The listing builds one solid part. Answer for the finished solid, in the listing's coordinates (mm). A direction names the side the tool comes from. Coordinates: 2 decimals unless noted, no trailing zeros. Order: outer loops, then holes, each group sorted by start corner. A loop starts at its lowest first (then second) coordinate and runs counter-clockwise, first axis right, second up.
```python
from build123d import *

# Parameters (mm, degrees)
ESQUISSE1_R                    = 1.25
ESQUISSE1_R_2                  = 5
BOSS_EXTRU_1_DEPTH             = 7.5
BOSS_EXTRU_2_DEPTH             = 40
BOSS_EXTRU_2_DIRECTION_2_REACH = 95.383
ESQUISSE4_W                    = 18
ESQUISSE4_H                    = 12.605144054
ENL_V_MAT_EXTRU_1_DEPTH        = 10
ENL_V_START                    = -7.5
ENL_V_MAT_EXTRU_2_DEPTH        = 7.5
BOSS_EXTRU_3_START             = -4
BOSS_EXTRU_3_DEPTH             = 4
BOSS_EXTRU_4_START             = -2
BOSS_EXTRU_4_DEPTH             = 2
ESQUISSE6_R                    = 1.5
ENL_V_MAT_EXTRU_3_DEPTH        = 10
ESQUISSE7_R                    = 3.1
ENL_V_MAT_EXTRU_4_DEPTH        = 2.5
ESQUISSE8_R                    = 3.6
ENL_V_MAT_EXTRU_5_DEPTH        = 0.7


with BuildPart() as part:
    # Esquisse1 → Boss.-Extru.1 (new body)
    with BuildSketch(Plane.XY):
        with BuildLine():
            ThreePointArc((23.75, 0), (0, 23.75), (-23.75, 0))
            Line((-23.75, 0), (-15, -75))
            ThreePointArc((-15, -75), (0, -90), (15, -75))
            Line((15, -75), (23.75, 0))
        make_face()
        with Locations((-5, 5)):
            Circle(ESQUISSE1_R, mode=Mode.SUBTRACT)
        with Locations((5, 5)):
            Circle(ESQUISSE1_R, mode=Mode.SUBTRACT)
        with Locations((5, -5)):
            Circle(ESQUISSE1_R, mode=Mode.SUBTRACT)
        with Locations((-5, -5)):
            Circle(ESQUISSE1_R, mode=Mode.SUBTRACT)
        with Locations((0, -75)):
            Circle(ESQUISSE1_R_2, mode=Mode.SUBTRACT)
    extrude(amount=BOSS_EXTRU_1_DEPTH)

    # Esquisse2 → Boss.-Extru.2 (add)
    with BuildSketch(Plane.XY.offset(7.5)):
        with BuildLine():
            ThreePointArc((-23.75, 0), (0, 23.75), (23.75, 0))
            Line((23.75, 0), (21.125, -22.5))
            Line((21.125, -22.5), (24.145347662, -22.5))
            Line((24.145347662, -22.5), (26.749397242, -0.17957503))
            ThreePointArc((26.749397242, -0.17957503), (0, 26.75), (-26.749397242, -0.17957503))
            Line((-26.749397242, -0.17957503), (-24.145347662, -22.5))
            Line((-24.145347662, -22.5), (-21.125, -22.5))
            Line((-21.125, -22.5), (-23.75, 0))
        make_face()
    extrude(amount=BOSS_EXTRU_2_DEPTH)

    # Boss.-Extru.2 direction 2: up to this face of the body (flat: up to its plane)
    boss_extru_2_direction_2_end = Plane(part.part.faces().sort_by_distance((0, -28.342449308, 0))[0])
    # Esquisse2 → Boss.-Extru.2 direction 2 (add, up to the picked face)
    with BuildSketch(Plane.XY.offset(7.5), mode=Mode.PRIVATE) as boss_extru_2_direction_2_sk1:
        with BuildLine():
            ThreePointArc((-23.75, 0), (0, 23.75), (23.75, 0))
            Line((23.75, 0), (21.125, -22.5))
            Line((21.125, -22.5), (24.145347662, -22.5))
            Line((24.145347662, -22.5), (26.749397242, -0.17957503))
            ThreePointArc((26.749397242, -0.17957503), (0, 26.75), (-26.749397242, -0.17957503))
            Line((-26.749397242, -0.17957503), (-24.145347662, -22.5))
            Line((-24.145347662, -22.5), (-21.125, -22.5))
            Line((-21.125, -22.5), (-23.75, 0))
        make_face()
    boss_extru_2_direction_2_tool1 = split(extrude(boss_extru_2_direction_2_sk1.sketch, amount=-BOSS_EXTRU_2_DIRECTION_2_REACH, mode=Mode.PRIVATE), bisect_by=boss_extru_2_direction_2_end, keep=Keep.BOTH, mode=Mode.PRIVATE)
    add(boss_extru_2_direction_2_tool1.solids().sort_by(Axis((0, 24.477173, 7.5), (0, 0, -1)))[0])

    # Esquisse4 → Enlèv. mat.-Extru.1 (cut)
    with BuildSketch(Plane.XY.offset(47.5)):
        with Locations((0, 26.75)):
            Rectangle(ESQUISSE4_W, ESQUISSE4_H)
    extrude(amount=-ENL_V_MAT_EXTRU_1_DEPTH, mode=Mode.SUBTRACT)

    # Esquisse5 → Enlèv. mat.-Extru.2 (cut)
    with BuildSketch(Plane.XY.offset(47.5).offset(ENL_V_START)):
        with BuildLine():
            Line((-11.411137634, 20.829028732), (-11.640060124, 21.354079473))
            Line((-11.640060124, 21.354079473), (-14.50858003, 21.678003669))
            Line((-14.50858003, 21.678003669), (-16.223366565, 19.355754657))
            Line((-16.223366565, 19.355754657), (-15.594359578, 17.913080398))
            ThreePointArc((-15.594359578, 17.913080398), (-13.581233692, 19.483649335), (-11.411137634, 20.829028732))
        make_face()
        Polygon((-21.820839715, -16.535659582), (-22.588746921, -16.571688322), (-23.913370218, -19.136587239), (-22.354414246, -21.566194123), (-21.240043834, -21.513909991), align=None)
    enl_v_mat_extru_2 = extrude(amount=ENL_V_MAT_EXTRU_2_DEPTH, mode=Mode.SUBTRACT)

    # Esquisse5<3> → Boss.-Extru.3 (add)
    with BuildSketch(Plane.XY.offset(47.5).offset(BOSS_EXTRU_3_START)):
        with BuildLine():
            ThreePointArc((-10.635661114, 21.235470625), (-11.025272446, 21.035823433), (-11.411137634, 20.829028732))
            Line((-11.411137634, 20.829028732), (-10.486326754, 18.707906265))
            Line((-10.486326754, 18.707906265), (-12.201113289, 16.385657254))
            Line((-12.201113289, 16.385657254), (-15.069633195, 16.70958145))
            Line((-15.069633195, 16.70958145), (-15.594359578, 17.913080398))
            ThreePointArc((-15.594359578, 17.913080398), (-15.976876587, 17.572760584), (-16.351968659, 17.224274178))
            ThreePointArc((-16.351968659, 17.224274178), (-12.416744053, 15.659892813), (-9.854846659, 19.031830461))
            ThreePointArc((-9.854846659, 19.031830461), (-10.055820333, 20.200772417), (-10.635661114, 21.235470625))
        make_face()
        with BuildLine():
            ThreePointArc((-17.529790949, -19.001295206), (-18.895919972, -16.227021489), (-21.927845037, -15.618471111))
            Line((-21.927845037, -15.618471111), (-21.820839715, -16.535659582))
            Line((-21.820839715, -16.535659582), (-19.705167652, -16.436396289))
            Line((-19.705167652, -16.436396289), (-18.14621168, -18.866003173))
            Line((-18.14621168, -18.866003173), (-19.470834977, -21.43090209))
            Line((-19.470834977, -21.43090209), (-21.240043834, -21.513909991))
            Line((-21.240043834, -21.513909991), (-21.125, -22.5))
            ThreePointArc((-21.125, -22.5), (-18.588810785, -21.509604565), (-17.529790949, -19.001295206))
        make_face()
    boss_extru_3 = extrude(amount=BOSS_EXTRU_3_DEPTH)

    # Esquisse5<4> → Boss.-Extru.4 (add)
    with BuildSketch(Plane.XY.offset(47.5).offset(BOSS_EXTRU_4_START)):
        with BuildLine():
            Line((-11.411137634, 20.829028732), (-11.640060124, 21.354079473))
            Line((-11.640060124, 21.354079473), (-14.50858003, 21.678003669))
            Line((-14.50858003, 21.678003669), (-16.223366565, 19.355754657))
            Line((-16.223366565, 19.355754657), (-15.594359578, 17.913080398))
            ThreePointArc((-15.594359578, 17.913080398), (-15.089714795, 18.340201945), (-14.573376801, 18.753111438))
            ThreePointArc((-14.573376801, 18.753111438), (-14.072849168, 20.055047153), (-12.678292605, 20.082913051))
            ThreePointArc((-12.678292605, 20.082913051), (-12.050491046, 20.465780355), (-11.411137634, 20.829028732))
        make_face()
        with BuildLine():
            Line((-10.486326754, 18.707906265), (-11.411137634, 20.829028732))
            ThreePointArc((-11.411137634, 20.829028732), (-12.050491046, 20.465780355), (-12.678292605, 20.082913051))
            ThreePointArc((-12.678292605, 20.082913051), (-12.257533448, 19.630498747), (-12.104846659, 19.031830461))
            ThreePointArc((-12.104846659, 19.031830461), (-13.214601654, 17.789722842), (-14.573376801, 18.753111438))
            ThreePointArc((-14.573376801, 18.753111438), (-15.089714795, 18.340201945), (-15.594359578, 17.913080398))
            Line((-15.594359578, 17.913080398), (-15.069633195, 16.70958145))
            Line((-15.069633195, 16.70958145), (-12.201113289, 16.385657254))
            Line((-12.201113289, 16.385657254), (-10.486326754, 18.707906265))
        make_face()
        with BuildLine():
            Line((-19.705167652, -16.436396289), (-21.820839715, -16.535659582))
            Line((-21.820839715, -16.535659582), (-21.659180538, -17.921309676))
            ThreePointArc((-21.659180538, -17.921309676), (-20.406989611, -17.917497027), (-19.779790949, -19.001295206))
            ThreePointArc((-19.779790949, -19.001295206), (-20.285594046, -20.005621333), (-21.393664499, -20.197161436))
            Line((-21.393664499, -20.197161436), (-21.240043834, -21.513909991))
            Line((-21.240043834, -21.513909991), (-19.470834977, -21.43090209))
            Line((-19.470834977, -21.43090209), (-18.14621168, -18.866003173))
            Line((-18.14621168, -18.866003173), (-19.705167652, -16.436396289))
        make_face()
        with BuildLine():
            Line((-21.659180538, -17.921309676), (-21.820839715, -16.535659582))
            Line((-21.820839715, -16.535659582), (-22.588746921, -16.571688322))
            Line((-22.588746921, -16.571688322), (-23.913370218, -19.136587239))
            Line((-23.913370218, -19.136587239), (-22.354414246, -21.566194123))
            Line((-22.354414246, -21.566194123), (-21.240043834, -21.513909991))
            Line((-21.240043834, -21.513909991), (-21.393664499, -20.197161436))
            ThreePointArc((-21.393664499, -20.197161436), (-22.271369873, -19.14614608), (-21.659180538, -17.921309676))
        make_face()
    boss_extru_4 = extrude(amount=BOSS_EXTRU_4_DEPTH)

    # Symétrie1: Enlèv. mat.-Extru.2, Boss.-Extru.3, Boss.-Extru.4 across plane
    add(enl_v_mat_extru_2.mirror(Plane(origin=(0, 0, 0), x_dir=(0, 0, 1), z_dir=(1, 0, 0))), mode=Mode.SUBTRACT)
    add(boss_extru_3.mirror(Plane(origin=(0, 0, 0), x_dir=(0, 0, 1), z_dir=(1, 0, 0))))
    add(boss_extru_4.mirror(Plane(origin=(0, 0, 0), x_dir=(0, 0, 1), z_dir=(1, 0, 0))))

    # Esquisse6 → Enlèv. mat.-Extru.3 (cut)
    with BuildSketch(Plane.XY.offset(7.5)):
        Circle(ESQUISSE6_R)
    extrude(amount=-ENL_V_MAT_EXTRU_3_DEPTH, mode=Mode.SUBTRACT)

    # Esquisse7 → Enlèv. mat.-Extru.4 (cut)
    with BuildSketch(Plane.XY.offset(7.5)):
        Circle(ESQUISSE7_R)
    extrude(amount=-ENL_V_MAT_EXTRU_4_DEPTH, mode=Mode.SUBTRACT)

    # Esquisse8 → Enlèv. mat.-Extru.5 (cut)
    with BuildSketch(Plane.XY.offset(7.5)):
        Circle(ESQUISSE8_R)
    extrude(amount=-ENL_V_MAT_EXTRU_5_DEPTH, mode=Mode.SUBTRACT)


solid = part.part
```
(1) Find section A-A (x = 0). Write down the section's boundary in (y, z), and give its area (3 significant figures).
(2) For faces 1 (the face through (3.434, 1.081, 7.155)), 2 (the face through (-9, 24, 43)), 3 (the face through (20, -20, 45.5)), 4 (the face through (18.02, -49.12, 3.7)), 5 (the face through (-5.27, 3.78, 3.7)), determine the directions among +Z, -Z, +X, -X, +Y, -Y from which every point of the face is accessible in a straight line to the end or side of a thin tool.
(3) The mould has two halves that part along Z. Classify faces 6 (the face through (-18, -20, 43.5)), 7 (the face through (1.43, -2.75, 5.91)), 8 (the face through (-24, 1, 47.5)): released by +Z, released by -Z, zero draft, split by the parting line, or undercut.
(4) Each of these flat-tipped pins is pushed along its axis until it touches: pin 1 Ø1 at (x, y) = (8, -42) entering from +Z; pin 2 Ø10 at (x, z) = (20, 13.5) entering from -Y; pin 3 Ø3.5 at (y, z) = (24.5, 43.5) entering from +X. Where does it stop, or does it pass through?
(5) Find section B-B (y = 5). Write down the section's boundary in (x, z), and give its area (3 significant figures).
(6) Consider line 1 (Y direction, x = 0, z = 6.4); line 2 (Z direction, x = 18.5, y = -17.5); line 3 (Z direction, x = 10.5, y = -49.5). Determine where each line is inside the solid, lowest interval first.
Findings below:
1. outline: (-90, 0) - (-80, 0) - (-80, 7.5) - (-90, 7.5) - close; (-70, 0) - (-1.5, 0) - (-1.5, 5) - (-3.1, 5) - (-3.1, 6.8) - (-3.6, 6.8) - (-3.6, 7.5) - (-70, 7.5) - close; (1.5, 0) - (26.75, 0) - (26.75, 37.5) - (23.75, 37.5) - (23.75, 7.5) - (3.6, 7.5) - (3.6, 6.8) - (3.1, 6.8) - (3.1, 5) - (1.5, 5) - close
1. area: 859 mm2
2. face 1: +Z
2. face 2: +Z, +Y, -Y
2. face 3: none
2. face 4: +Z, -Z, +X, -Y
2. face 5: +Z, -Z
3. face 6: undercut
3. face 7: zero draft
3. face 8: released by +Z
4. pin 1: stops at z = 7.5
4. pin 2: stops at y = -22.5
4. pin 3: stops at x = 14.07
5. outline: (-26.28, 0) - (-6.25, 0) - (-6.25, 7.5) - (-23.22, 7.5) - (-23.22, 47.5) - (-26.28, 47.5) - close; (-3.75, 0) - (3.75, 0) - (3.75, 7.5) - (-3.75, 7.5) - close; (6.25, 0) - (26.28, 0) - (26.28, 47.5) - (23.22, 47.5) - (23.22, 7.5) - (6.25, 7.5) - close
5. area: 602 mm2
6. line 1: y = -90 to -80, -70 to -3.1, 3.1 to 26.75
6. line 2: z = 0 to 7.5, 43.5 to 47.5
6. line 3: z = 0 to 7.5
